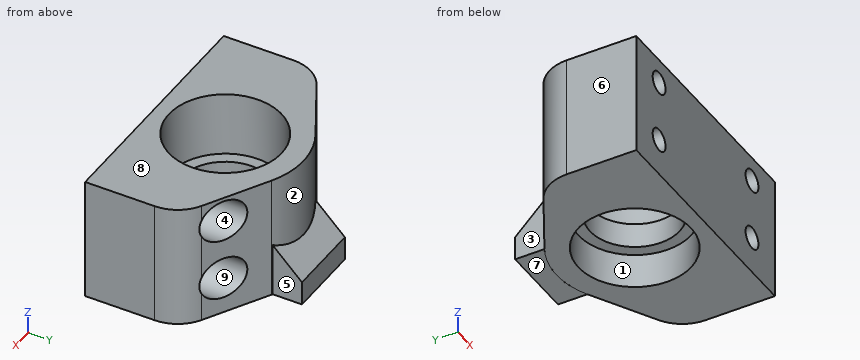
from build123d import *

# Parameters (mm, degrees)
SKETCH1_R           = 9
BOSS_EXTRUDE1_DEPTH = 25
SKETCH2_R           = 11.335
CUT_EXTRUDE1_DEPTH  = 13
CUT_EXTRUDE2_START  = -7
SKETCH3_R           = 11.335
CUT_EXTRUDE2_DEPTH  = 7
BOSS_EXTRUDE2_DEPTH = 4.85
BOSS_EXTRUDE3_DEPTH = 15
SKETCH6_R           = 2.25
CUT_EXTRUDE3_DEPTH  = 49.673016138
SKETCH7_R           = 4.25
CUT_EXTRUDE4_DEPTH  = 43.297310789


with BuildPart() as part:
    # Sketch1 → Boss-Extrude1 (new body)
    with BuildSketch(Plane.XY):
        with BuildLine():
            Line((24.25, 4), (24.25, -10))
            Line((24.25, -10), (-24.25, -10))
            Line((-24.25, -10), (-24.25, 4))
            ThreePointArc((-24.25, 4), (-23.13858198, 8.090248735), (-20.11, 11.055560845))
            Line((-20.11, 11.055560845), (-7.682261614, 17.999376585))
            ThreePointArc((-7.682261614, 17.999376585), (0, 20), (7.682261614, 17.999376585))
            Line((7.682261614, 17.999376585), (20.11, 11.055560845))
            ThreePointArc((20.11, 11.055560845), (23.13858198, 8.090248735), (24.25, 4))
        make_face()
        with Locations((0, 4.25)):
            Circle(SKETCH1_R, mode=Mode.SUBTRACT)
    extrude(amount=BOSS_EXTRUDE1_DEPTH)

    # Sketch2 → Cut-Extrude1 (cut)
    with BuildSketch(Plane.XY.offset(25)):
        with Locations((0, 4.25)):
            Circle(SKETCH2_R)
    extrude(amount=-CUT_EXTRUDE1_DEPTH, mode=Mode.SUBTRACT)

    # Sketch3 → Cut-Extrude2 (cut)
    with BuildSketch(Plane(origin=(0, 0, 0), x_dir=(-1, 0, 0), z_dir=(0, 0, -1)).offset(CUT_EXTRUDE2_START)):
        with Locations(Location((0, 4.25, 0), (0, 0, 180))):
            Circle(SKETCH3_R)
    extrude(amount=CUT_EXTRUDE2_DEPTH, mode=Mode.SUBTRACT)



with BuildPart() as body_2:
    # Sketch4 → Boss-Extrude2 (new body)
    with BuildSketch(Plane(origin=(0, 0, 0), x_dir=(-1, 0, 0), z_dir=(0, 0, -1))):
        with BuildLine():
            Line((-7.5, 18.101212577), (-7.5, 24))
            Line((-7.5, 24), (7.5, 24))
            Line((7.5, 24), (7.5, 18.101212577))
            ThreePointArc((7.5, 18.101212577), (0, 20.001383744), (-7.5, 18.101212577))
        make_face()
    extrude(amount=-BOSS_EXTRUDE2_DEPTH)


with BuildPart() as part_1:
    add(part.part)

    add(body_2.part)  # Boss-Extrude3 merges body 2
    # Sketch5 → Boss-Extrude3 (add)
    with BuildSketch(Plane(origin=(7.5, 0, 0), x_dir=(0, 0, -1), z_dir=(1, 0, 0))):
        Polygon((-4.85, 24), (-4.85, 18.101212577), (-10.748787423, 18.101212577), align=None)
    extrude(amount=-BOSS_EXTRUDE3_DEPTH)

    # Sketch6 → Cut-Extrude3 (cut, through all)
    with BuildSketch(Plane.XZ.offset(10)):
        with Locations((-16.25, 20)):
            Circle(SKETCH6_R)
        with Locations((16.25, 20)):
            Circle(SKETCH6_R)
        with Locations((16.25, 7.5)):
            Circle(SKETCH6_R)
        with Locations((-16.25, 7.5)):
            Circle(SKETCH6_R)
    extrude(amount=-CUT_EXTRUDE3_DEPTH, mode=Mode.SUBTRACT)

    # Sketch7 → Cut-Extrude4 (cut, through all)
    with BuildSketch(Plane(origin=(0, 0, 0), x_dir=(-1, 0, 0), z_dir=(0, -1, 0))):
        with Locations(Location((16.25, -20, 0), (0, 0, 180))):
            Circle(SKETCH7_R)
        with Locations(Location((16.25, -7.5, 0), (0, 0, 180))):
            Circle(SKETCH7_R)
        with Locations(Location((-16.25, -7.5, 0), (0, 0, 180))):
            Circle(SKETCH7_R)
        with Locations(Location((-16.25, -20, 0), (0, 0, 180))):
            Circle(SKETCH7_R)
    extrude(amount=-CUT_EXTRUDE4_DEPTH, mode=Mode.SUBTRACT)


solid = part_1.part
For this review, take the finished solid that the model builds, in its own axes (mm). Face numbers are marked on the shaded views. A direction names the side the tool comes from. Coordinates: 2 decimals unless noted, no trailing zeros. Write each loop counter-clockwise with the first axis right and the second up, starting at its lowest first coordinate (ties: lowest second). Pieces come first, ordered by that corner, then holes. Notation, with made-up numbers: (28.5, 37.25) -> (47.5, 37.25) arc R6 ccw to (47.5, 41.25) -> close; hole circle Ø6 at (14, 42). An arc over 180 degrees is marked (long way). Write each question's results on one line, items separated by ' | '. Start each with the question number.
1) The part is to be moulded in two halves that separate along Z. For the marked faces 6, 7, 8 and 9, say which applies: +Z half, -Z half, draft (parallel to the pull), parting line (faces both ways), or undercut.
2) For the marked faces 1, 2, 3, 4 and 5, list the 3-axis set-ups (+Z, -Z, +X, -X, +Y, -Y) from which the entire face can be reached by the end or side of a thin tool; tool diameter is ignored.
3) Wall thickness on L1, parallel to Z at x = 16, y = 10; L2, parallel to Y at x = 0, z = 21.5 (3 decimals); L3, parallel to X at y = -4.5, z = 6.25: over which ranges is each line inside the solid? List them lowest first. Write a range as [from, to].
4) Consider section A-A (z = 2.5). Write out the cut boundary in (x, y) (3 decimals), plus the area to 3 significant figures.
5) Insertion check: pin 1 (7 mm diameter, centred on x = -14, z = 8.5, fed in from +Y) (3 decimals); pin 2 (4 mm diameter, centred on x = 17.5, z = 20, fed in from +Y); pin 3 (5 mm diameter, centred on y = 9, z = 13, fed in from -X); pin 4 (16 mm diameter, centred on x = 0, y = 4.25, fed in from -Z). Each pin has a flat end and moves straight along its axis. Give the tip position at first contact, or say it passes through.
6) Consider section C-C (z = 14.75). Write out the cut boundary in (x, y) (3 decimals).
7) Consider section D-D (x = -17). Write out the cut boundary in (y, z), plus the area to 3 significant figures.
Geometry says:
1) face 6: draft | face 7: -Z half | face 8: +Z half | face 9: undercut
2) face 1: -Z | face 2: none | face 3: +Z, -Z, -X, +Y | face 4: +Y | face 5: +Z, -Z, +X, +Y
3) L1: [0, 3.26], [11.74, 15.76], [24.24, 25] | L2: [-10, -7.085], [15.585, 20] | L3: [-24.25, -18.12], [-14.38, -7.21], [7.21, 14.38], [18.12, 24.25]
4) outline: (-24.25, -10) -> (24.25, -10) -> (24.25, 4) arc R8.082 ccw to (20.11, 11.056) -> (7.682, 17.999) arc R15.75 ccw to (-7.682, 17.999) -> (-20.11, 11.056) arc R8.082 ccw to (-24.25, 4) -> close; (-7.5, 18.101) arc R15.751 cw to (7.5, 18.101) -> (7.5, 24) -> (-7.5, 24) -> close; hole circle Ø22.67 at (0, 4.25) | area: 884 mm^2
5) pin 1: y = 16.425 | pin 2: y = 0 | pin 3: x = -23.85 | pin 4: through
6) outline: (-24.25, -10) -> (24.25, -10) -> (24.25, 4) arc R8.082 ccw to (20.11, 11.056) -> (7.682, 17.999) arc R15.75 ccw to (-7.682, 17.999) -> (-20.11, 11.056) arc R8.082 ccw to (-24.25, 4) -> close; hole circle Ø22.67 at (0, 4.25)
7) outline: (-10, 0) -> (12.79, 0) -> (12.79, 3.32) -> (0, 3.32) -> (0, 5.38) -> (-10, 5.38) -> close; (-10, 9.62) -> (0, 9.62) -> (0, 11.68) -> (12.79, 11.68) -> (12.79, 15.82) -> (0, 15.82) -> (0, 17.88) -> (-10, 17.88) -> close; (-10, 22.12) -> (0, 22.12) -> (0, 24.18) -> (12.79, 24.18) -> (12.79, 25) -> (-10, 25) -> close | area: 271 mm^2
